Geometry: see drawing. Coordinates: mm, zero at the bounding-box minimum. A direction names the side the tool comes from. Coordinates: 2 decimals unless noted, no trailing zeros. Write each loop counter-clockwise with the first axis right and the second up, starting at its lowest first coordinate (ties: lowest second). Pieces come first, ordered by that corner, then holes. Notation, with made-up numbers: (-38.5, 85) - (20.5, 85) arc R16 ccw to (20.5, 111) - close; hole circle Ø9 at (40.5, -25.75). An arc over 180 degrees is marked (long way). Use a Markdown table: item, result. Add a question column.
Q1. Material intervals for probe 1 along Z at (x, y) = (11.75, 8); probe 2 along X at (y, z) = (3.25, 12.5), sorted ascending. Write a range as from..to.
Q2. Pin query (flat end, axial travel): P1, Ø8, axis at x = 12.5, y = 5, coming from the +Z side; P2, Ø4, axis at x = 10.5, y = 12, coming from the +Z side; P3, Ø1, axis at x = 5.5, z = 4, coming from the +Y side. Return the tip coordinate at first contact, or that it passes through.
Q3. Section query C-C (x = 13.75). Return the cut outline in (y, z).
Q4. Section query A-A (y = 8). Return the cut outline in (x, z), then the cut area to 3 significant figures.
Q5. Mould query, pull axis X, two halves, no side actions, for the marked faces 1, 2, 3 and 4. Classes: released by +X, released by -X, zero draft, split by the parting line, or undercut.
Q6. Set-up query: the marked faces 5 and 6. Return all of +Z, -Z, +X, -X, +Y, -Y with unobstructed straight access to the full face (end or side cutting, diameter ignored); none if empty.
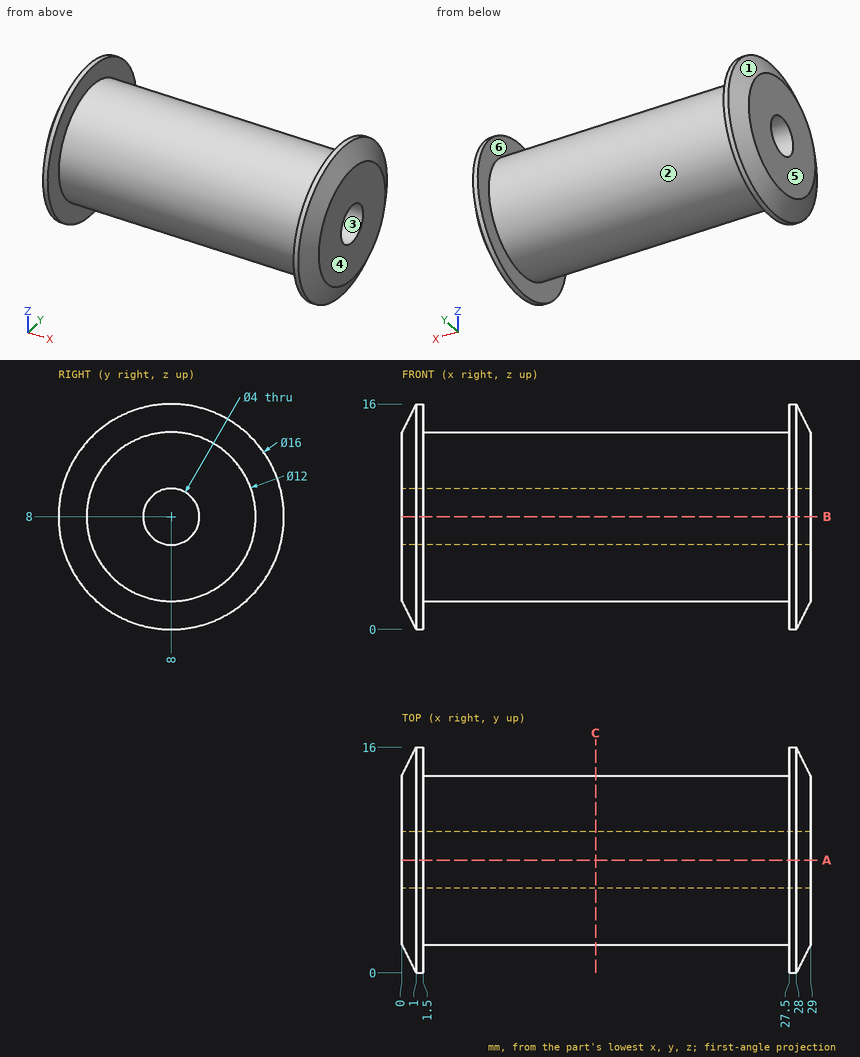
Values follow:
| question | item | result |
|---|---|---|
| 1 | probe 1 | 2..6, 10..14 |
| 1 | probe 2 | 0.27..1.5, 27.5..28.73 |
| 2 | P1 | z = 14 |
| 2 | P2 | z = 13.66 |
| 2 | P3 | y = 12.87 |
| 3 | outline | circle Ø12 at (8, 8); hole circle Ø4 at (8, 8) |
| 4 | outline | (0, 2) - (1, 0) - (1.5, 0) - (1.5, 2) - (27.5, 2) - (27.5, 0) - (28, 0) - (29, 2) - (29, 6) - (0, 6) - close; (0, 10) - (29, 10) - (29, 14) - (28, 16) - (27.5, 16) - (27.5, 14) - (1.5, 14) - (1.5, 16) - (1, 16) - (0, 14) - close |
| 4 | area | 240 mm2 |
| 5 | face 1 | released by -X |
| 5 | face 2 | undercut |
| 5 | face 3 | zero draft |
| 5 | face 4 | released by +X |
| 6 | face 5 | +Z, -Z, -X, +Y, -Y |
| 6 | face 6 | none |
